```python
from build123d import *

# Parameters (mm, degrees)
ESQUISSE1_R             = 2.5
BOSS_EXTRU_1_DEPTH      = 30
CHANFREIN1_SIZE         = 2
CONG_2_R                = 1
ENL_V_MAT_EXTRU_1_DEPTH = 10
ENL_V_START             = -10
ENL_V_MAT_EXTRU_2_DEPTH = 10
ENL_V_MAT_EXTRU_3_DEPTH = 53.665216263
CONG_3_R                = 1
CONG_4_R                = 4


with BuildPart() as part:
    # Esquisse1 → Boss.-Extru.1 (new body)
    with BuildSketch(Plane.XY):
        with BuildLine():
            Line((13.4187369, 3), (16.479153498, 3))
            ThreePointArc((16.479153498, 3), (10.731088016, 12.861036117), (0, 16.75))
            Line((0, 16.75), (-45.75, 16.75))
            Line((-45.75, 16.75), (-45.75, -16.75))
            Line((-45.75, -16.75), (0, -16.75))
            ThreePointArc((0, -16.75), (10.731088016, -12.861036117), (16.479153498, -3))
            Line((16.479153498, -3), (13.4187369, -3))
            ThreePointArc((13.4187369, -3), (-13.75, 0), (13.4187369, 3))
        make_face()
        with Locations((-37, 0)):
            Circle(ESQUISSE1_R, mode=Mode.SUBTRACT)
        with Locations((-27, 0)):
            Circle(ESQUISSE1_R, mode=Mode.SUBTRACT)
    extrude(amount=BOSS_EXTRU_1_DEPTH)

    # Chanfrein1
    chanfrein1_edges = [part.edges().sort_by_distance(p)[0] for p in [
        (-13.75, 0, 0),
    ]]
    chamfer(chanfrein1_edges, length=CHANFREIN1_SIZE)

    # Congé2
    # the kernel refuses this fillet: 1 mm, written as the material it takes off along each edge
    with BuildSketch(Plane(origin=(16.479153498, -3, -3.211221849), x_dir=(-1, 0, 0), z_dir=(0, 0, 1))) as cong_2_piece_1:
        with BuildLine():
            CenterArc((1.245555761, 1), CONG_2_R, 165.287542039, 104.712457961)
            ThreePointArc((0.278343206, 1.253968254), (0.127146972, 0.629653233), (0, 0))
            Line((0, 0), (1.245555761, 0))
        make_face()
    extrude(amount=36.422443699, mode=Mode.SUBTRACT)
    with BuildSketch(Plane(origin=(16.479153498, 3, -3.211221849), x_dir=(-1, 0, 0), z_dir=(0, 0, 1))) as cong_2_piece_2:
        with BuildLine():
            CenterArc((1.245555761, -1), CONG_2_R, 90, 104.712457961)
            ThreePointArc((0.278343206, -1.253968254), (0.127146972, -0.629653233), (0, 0))
            Line((0, 0), (1.245555761, 0))
        make_face()
    extrude(amount=36.422443699, mode=Mode.SUBTRACT)
    with BuildSketch(Plane(origin=(13.4187369, -3, 0.05366509), x_dir=(1, 0, 0), z_dir=(0, 0, 1))) as cong_2_piece_3:
        with BuildLine():
            CenterArc((0.778533964, -1), CONG_2_R, 90, 74.265120821)
            ThreePointArc((-0.183992874, -0.728813559), (-0.087015193, -0.365664321), (0, 0))
            Line((0, 0), (0.778533964, 0))
        make_face()
    extrude(amount=31.892669821, mode=Mode.SUBTRACT)
    with BuildSketch(Plane(origin=(13.4187369, 3, 0.05366509), x_dir=(-0.24477558700132723, 0.9695797605190384, 0), z_dir=(0, 0, 1))) as cong_2_piece_4:
        with BuildLine():
            CenterArc((0.779013652, -0.999626362), CONG_2_R, 91.566307169, 74.265120821)
            Line((-0.190566108, -0.754850775), (0, 0))
            ThreePointArc((0, 0), (0.37583992, -0.005137529), (0.75167984, 0))
        make_face()
    extrude(amount=31.892669821, mode=Mode.SUBTRACT)

    # Esquisse2 → Enlèv. mat.-Extru.1 (cut)
    with BuildSketch(Plane(origin=(0, 0, 0), x_dir=(-1, 0, 0), z_dir=(0, 0, -1))):
        with BuildLine():
            Line((45.75, 10.1), (27, 10.1))
            ThreePointArc((27, 10.1), (16.9, 0), (27, -10.1))
            Line((27, -10.1), (45.75, -10.1))
            Line((45.75, -10.1), (45.75, 10.1))
        make_face()
    extrude(amount=-ENL_V_MAT_EXTRU_1_DEPTH, mode=Mode.SUBTRACT)

    # Esquisse3 → Enlèv. mat.-Extru.2 (cut)
    with BuildSketch(Plane.XY.offset(30).offset(ENL_V_START)):
        with BuildLine():
            Line((0, 16.75), (-45.75, 16.75))
            Line((-45.75, 16.75), (-45.75, -16.75))
            Line((-45.75, -16.75), (0, -16.75))
            ThreePointArc((0, -16.75), (-16.75, 0), (0, 16.75))
        make_face()
    extrude(amount=ENL_V_MAT_EXTRU_2_DEPTH, mode=Mode.SUBTRACT)

    # Esquisse5 → Enlèv. mat.-Extru.3 (cut, through all)
    with BuildSketch(Plane.XY.offset(20)):
        Polygon((-15.75, 16.75), (-45.75, 9.75), (-45.75, 16.75), align=None)
        Polygon((-45.75, -16.75), (-15.75, -16.75), (-45.75, -9.75), align=None)
    extrude(amount=-ENL_V_MAT_EXTRU_3_DEPTH, mode=Mode.SUBTRACT)

    # Congé3
    cong_3_edges = [part.edges().sort_by_distance(p)[0] for p in [
        (-44.25, 10.1, 5),
        (-44.25, -10.1, 5),
    ]]
    fillet(cong_3_edges, radius=CONG_3_R)

    # Congé4
    cong_4_edges = [part.edges().sort_by_distance(p)[0] for p in [
        (-45.75, 9.75, 15),
        (-45.75, -9.75, 15),
    ]]
    fillet(cong_4_edges, radius=CONG_4_R)


solid = part.part
```
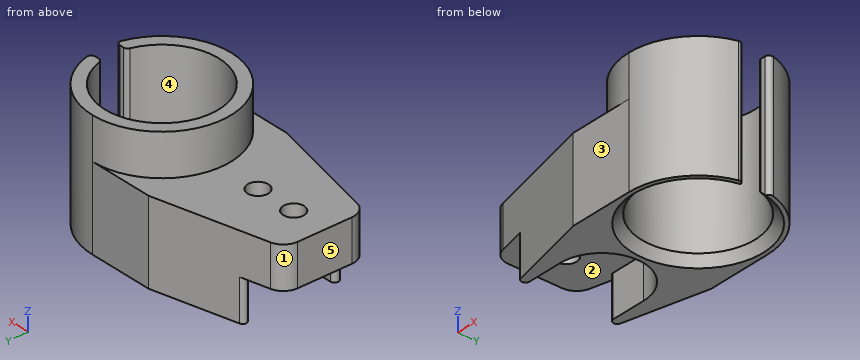
Check sheet for the modelled part. Datum: model origin and axes. Units: mm. Face numbers are marked on the shaded views. A direction names the side the tool comes from. Give positions to 0.01 mm unless a question says otherwise; leave off trailing zeros. Order: outer loops, then holes, each group sorted by start corner. A loop starts at its lowest first (then second) coordinate and runs counter-clockwise, first axis right, second up. Notation, with made-up numbers: M 61,59.25 L 74,59.25 A19 ccw 74,89.25 Z; hole C -16,-30.75 d9. An arc over 180 degrees is marked long. Answer in a Markdown table with one row per item.
1) Gauge pin test, flat ends, axial feed: P1, Ø1.5, axis at x = -14.5, y = 2.5, coming from the -Z side; P2, Ø8, axis at x = -27, y = 0, coming from the +Z side; P3, Ø4, axis at x = -19, z = 14.5, coming from the +Y side. Record the tip position at first contact, or that the pin passes through.
Filled sheet:
| item | result |
|---|---|
| P1 | stops at z = 0.29 |
| P2 | stops at z = 20 |
| P3 | stops at y = 16.46 |
2) Thickness scan on L1, parallel to Y at x = -20, z = 16.5; L2, parallel to Z at x = -15, y = -12.5; L3, parallel to Y at x = -37, z = 13.25. Record the ranges inside material, lowest first. Write a range as [from, to].
Filled sheet:
| item | result |
|---|---|
| L1 | y = [-15.76, 15.76] |
| L2 | z = [0, 20] |
| L3 | y = [-11.79, -2.5], [2.5, 11.79] |
3) Cross-section at C-C, the plane x = -25.5. Enter the section's corners in (y, z) (3 decimals).
Filled sheet:
| item | result |
|---|---|
| outline | M -14.475,0 L -9.988,0 L -9.988,10 L -2,10 L -2,20 L -14.475,20 Z; M 2,10 L 9.988,10 L 9.988,0 L 14.475,0 L 14.475,20 L 2,20 Z |
4) Access from +Z, -Z, +X, -X, +Y, -Y to the whole of each face (thin tool, end or side, straight path). Record for the marked faces 1 and 2.
Filled sheet:
| item | result |
|---|---|
| face 1 | +Z, -Z, -X, +Y |
| face 2 | -Z, -X |
5) Cross-section at B-B, the plane y = 0. Enter the section's corners in (x, z).
Filled sheet:
| item | result |
|---|---|
| outline | M -45.75,10 L -39.5,10 L -39.5,20 L -45.75,20 Z; M -34.5,10 L -29.5,10 L -29.5,20 L -34.5,20 Z; M -24.5,10 L -16.9,10 L -16.9,0 L -15.75,0 L -13.75,2 L -13.75,30 L -16.75,30 L -16.75,20 L -24.5,20 Z |
6) Cross-section at D-D, the plane z = 24.5. Enter the section's corners in (x, y).
Filled sheet:
| item | result |
|---|---|
| outline | M 13.23,-3.73 A13.75 cw long 13.23,3.73 A1 ccw 14.2,3 L 15.23,3 A1 ccw 16.2,4.25 A16.75 ccw long 16.2,-4.25 A1 ccw 15.23,-3 L 14.2,-3 A1 ccw Z |
7) Cross-section at A-A, the plane z = 17.5. Enter the section's corners in (x, y).
Filled sheet:
| item | result |
|---|---|
| outline | M -45.75,-6.58 A4 ccw -42.66,-10.47 L -15.75,-16.75 L 0,-16.75 A16.75 ccw 16.2,-4.25 A1 ccw 15.23,-3 L 14.2,-3 A1 ccw 13.23,-3.73 A13.75 cw long 13.23,3.73 A1 ccw 14.2,3 L 15.23,3 A1 ccw 16.2,4.25 A16.75 ccw 0,16.75 L -15.75,16.75 L -42.66,10.47 A4 ccw -45.75,6.58 Z; hole C -37,0 d5; hole C -27,0 d5 |
8) Release check for a two-part mould opening along Y. For the marked faces 3, 4 and 5 record: +Y half, -Y half, draft (parallel to the pull), parting line (faces both ways), or undercut.
Filled sheet:
| item | result |
|---|---|
| face 3 | -Y half |
| face 4 | undercut |
| face 5 | draft |
